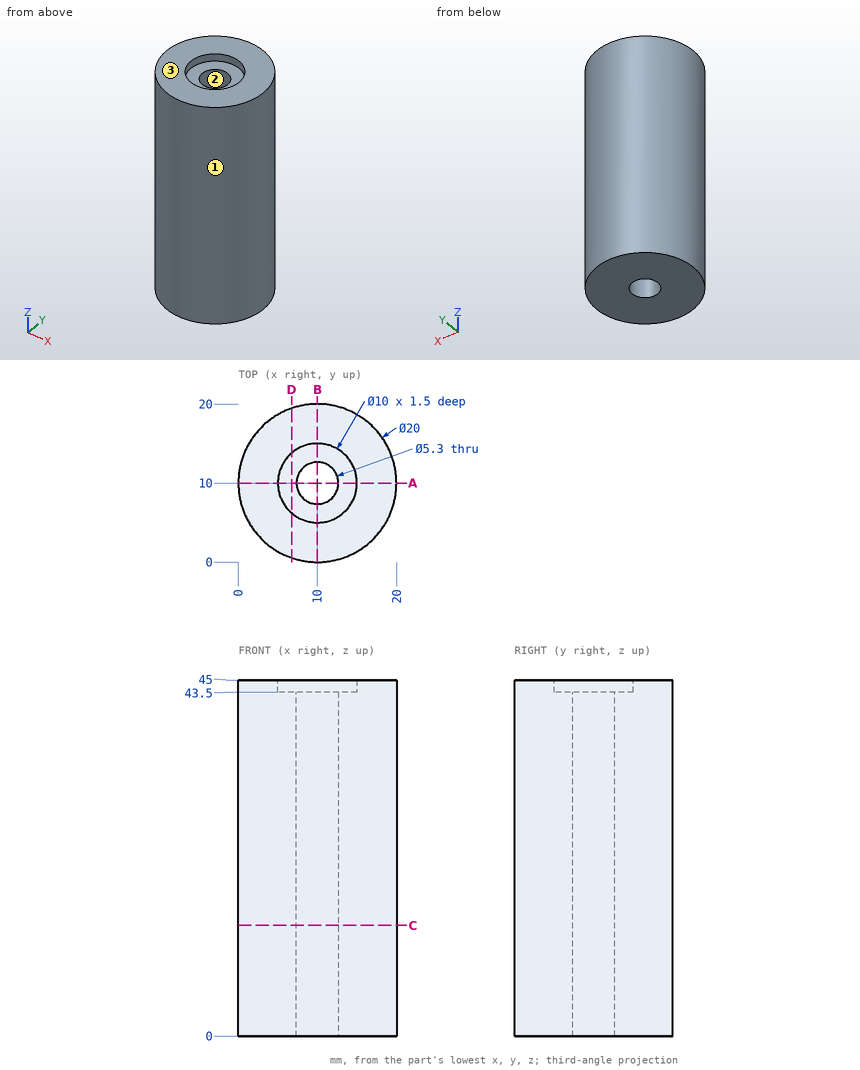
Answer from the drawing. Dimensions are ordinates in mm from the lowest x, y and z of the part. Coordinates: 2 decimals unless noted, no trailing zeros. Order: outer loops, then holes, each group sorted by start corner. A loop starts at its lowest first (then second) coordinate and runs counter-clockwise, first axis right, second up. Notation, with made-up numbers: M -14.5,30.5 L 16.5,30.5 A6 ccw 16.5,40.5 Z; hole C 33,-39 d7. An arc over 180 degrees is marked long. Put each result on its own line as item: value. Start each with the question number.
Item 1: The mould has two halves that part along X. Classify the marked faces 1, 2 and 3: +X half, -X half, draft (parallel to the pull), parting line (faces both ways), or undercut.
Item 2: Section A-A, the plane y = 10 is taken. Determine the outline of the cut face in (x, z).
Item 3: Given pin 1 Ø5 at (y, z) = (15, 31) entering from -X; pin 2 Ø3 at (x, y) = (11, 10) entering from +Z; pin 3 Ø1 at (x, z) = (17, 38.5) entering from +Y; pin 4 Ø8 at (x, y) = (10, 10) entering from +Z, each flat-ended and moving along its own axis, determine where each tip first touches the part or whether it passes through.
Item 4: Section C-C, the plane z = 14 is taken. Determine the outline of the cut face in (x, y).
Item 5: Consider probe 1 along Y at (x, z) = (10, 32.5); probe 2 along Y at (x, z) = (10, 44.2); probe 3 along Z at (x, y) = (11.5, 12.25). Determine where each line is inside the solid, lowest interval first. Write a range as [from, to].
Item 6: Section D-D, the plane x = 6.75 is taken. Determine the outline of the cut face in (y, z), plus the area to 3 significant figures.
Computed:
1. face 1: parting line
1. face 2: undercut
1. face 3: draft
2. outline: M 0,0 L 7.35,0 L 7.35,43.5 L 5,43.5 L 5,45 L 0,45 Z; M 12.65,0 L 20,0 L 20,45 L 15,45 L 15,43.5 L 12.65,43.5 Z
3. pin 1: stops at x = 0.32
3. pin 2: passes through
3. pin 3: stops at y = 17.6
3. pin 4: stops at z = 43.5
4. outline: C 10,10 d20; hole C 10,10 d5.3
5. probe 1: y = [0, 7.35], [12.65, 20]
5. probe 2: y = [0, 5], [15, 20]
5. probe 3: z = [0, 43.5]
6. outline: M 0.54,0 L 19.46,0 L 19.46,45 L 13.8,45 L 13.8,43.5 L 6.2,43.5 L 6.2,45 L 0.54,45 Z
6. area: 840 mm2
